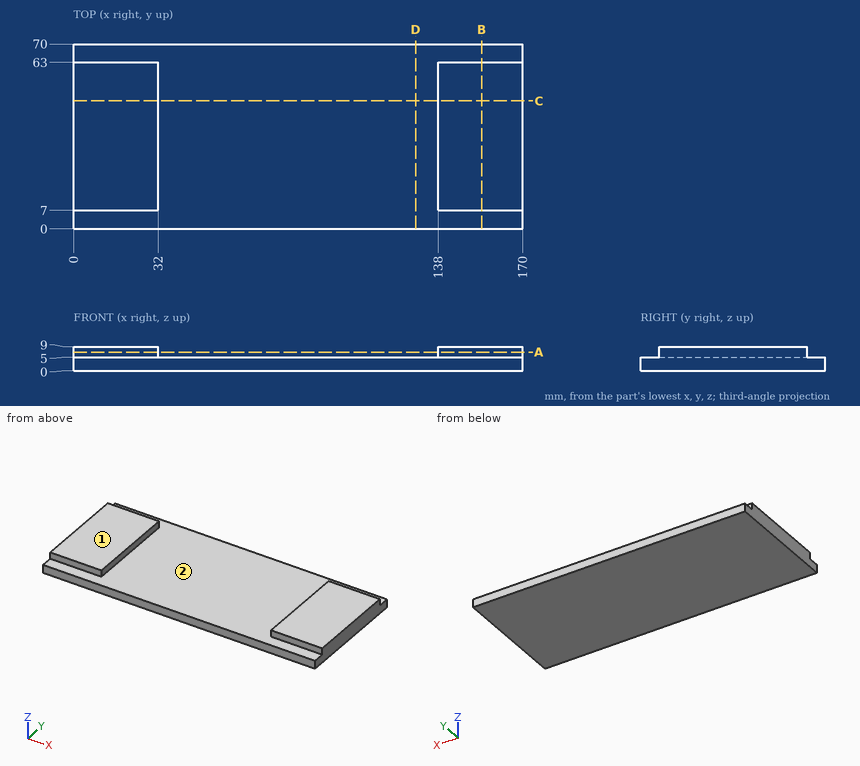
Answer from the drawing. Dimensions are ordinates in mm from the lowest x, y and z of the part. Coordinates: 2 decimals unless noted, no trailing zeros. Loops run counter-clockwise (first coordinate to the right, second up) from the corner with the lowest first, then second, coordinate; pieces in that order, holes last.
Q1. Consider probe 1 along X at (y, z) = (21, 7); probe 2 along Z at (x, y) = (100, 49.5); probe 3 along Y at (x, z) = (10.5, 5.5). Determine where each line is inside the solid, lowest interval first.
Q2. The part is cut by section D-D on x = 129.5. Write down the section's boundary in (y, z).
Q3. The part is cut by section B-B on x = 154.5. Write down the section's boundary in (y, z), and give its area (3 significant figures).
Q4. The part is cut by section A-A on z = 7. Write down the section's boundary in (x, y).
Q5. The mould has two halves that part along X. Classify the marked faces 1 and 2: +X half, -X half, draft (parallel to the pull), parting line (faces both ways), or undercut.
Q6. The part is cut by section C-C on y = 48.5. Write down the section's boundary in (x, z), and give its area (3 significant figures).
Q7. Each of these flat-tipped pins is pushed along its axis until it touches: pin 1 Ø2 at (x, z) = (12.5, 6.5) entering from -Y; pin 2 Ø1 at (x, z) = (40.5, 6) entering from -Y; pin 3 Ø21 at (x, y) = (84.5, 23) entering from +Z. Where does it stop, or does it pass through?
Results below:
1. probe 1: x = 0 to 32, 138 to 170
1. probe 2: z = 0 to 5
1. probe 3: y = 7 to 63
2. outline: (0, 0) - (70, 0) - (70, 5) - (0, 5) - close
3. outline: (0, 0) - (70, 0) - (70, 5) - (63, 5) - (63, 9) - (7, 9) - (7, 5) - (0, 5) - close
3. area: 574 mm2
4. outline: (0, 7) - (32, 7) - (32, 63) - (0, 63) - close; (138, 7) - (170, 7) - (170, 63) - (138, 63) - close
5. face 1: draft
5. face 2: undercut
6. outline: (0, 0) - (170, 0) - (170, 9) - (138, 9) - (138, 5) - (32, 5) - (32, 9) - (0, 9) - close
6. area: 1,110 mm2
7. pin 1: stops at y = 7
7. pin 2: passes through
7. pin 3: stops at z = 5
